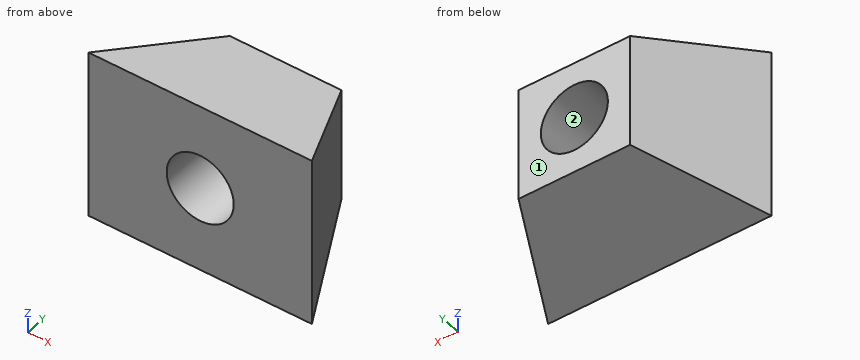
```python
from build123d import *

# Parameters (mm, degrees)
HOLE_FOR_HOOK_START     = -12.7
HOLE_FOR_HOOK_OUTLINE_R = 3.81
HOLE_FOR_HOOK_DEPTH     = 12.7


# Read off the part's stored shape, not the designer's step: Hole-For-Hook
with BuildPart() as part:
    # Sketch-Rectangle → Loft1 section 0
    with BuildSketch(Plane(origin=(0, 0, 0), x_dir=(1, 0, 0), z_dir=(0, 1, 0))):
        with BuildLine():
            Line((-12.7, -9.525), (12.7, -9.525))
            Line((12.7, -9.525), (12.7, 9.525))
            Line((12.7, 9.525), (-12.7, 9.525))
            Line((-12.7, 9.525), (-12.7, -9.525))
        make_face()
    # Sketch-Square → Loft1 section 1
    with BuildSketch(Plane(origin=(0, 12.7, 0), x_dir=(1, 0, 0), z_dir=(0, 1, 0))):
        with BuildLine():
            Line((-6.35, -6.35), (6.35, -6.35))
            Line((6.35, -6.35), (6.35, 6.35))
            Line((6.35, 6.35), (-6.35, 6.35))
            Line((-6.35, 6.35), (-6.35, -6.35))
        make_face()
    loft()

    # Hole-For-Hook outline → Hole-For-Hook (cut)
    with BuildSketch(Plane(origin=(0, 12.7, 0), x_dir=(1, 0, 0), z_dir=(0, 1, 0)).offset(HOLE_FOR_HOOK_START)):
        Circle(HOLE_FOR_HOOK_OUTLINE_R)
    extrude(amount=HOLE_FOR_HOOK_DEPTH, mode=Mode.SUBTRACT)


solid = part.part
```
Could you check a few things on this model? Use its own coordinates, in mm. Face numbers are marked on the shaded views. Round coordinates to 2 decimals unless told otherwise and drop trailing zeros. One line per question, with ' | ' between items. Start each with the question number.
(1) Thinking about a two-plate mould opening in Z: for the marked faces 1 and 2, which applies, +Z half, -Z half, draft (parallel to the pull), parting line (faces both ways), or undercut?
(2) Please list where these lines run through material, in increasing order: line 1 along Z through (x, y) = (0, 6) (3 decimals); line 2 along Z through (x, y) = (0, 8.25); line 3 along X through (y, z) = (4, 0).
(3) For P1, Ø6, axis at y = 4.5, z = -5.5, coming from the -X side; P2, Ø6, axis at y = 2, z = -6.5, coming from the +X side; P3, Ø6, axis at y = 5, z = -6.5, coming from the -X side, each with a flat end and sliding along its axis, tell me the tip position at first contact or that it passes through.
Geometry results:
1) face 1: draft | face 2: undercut
2) line 1: -8.025 to -3.81, 3.81 to 8.025 | line 2: -7.46 to -3.81, 3.81 to 7.46 | line 3: -10.7 to -3.81, 3.81 to 10.7
3) P1: x = -11.95 | P2: x = 12.7 | P3: x = -11.7
